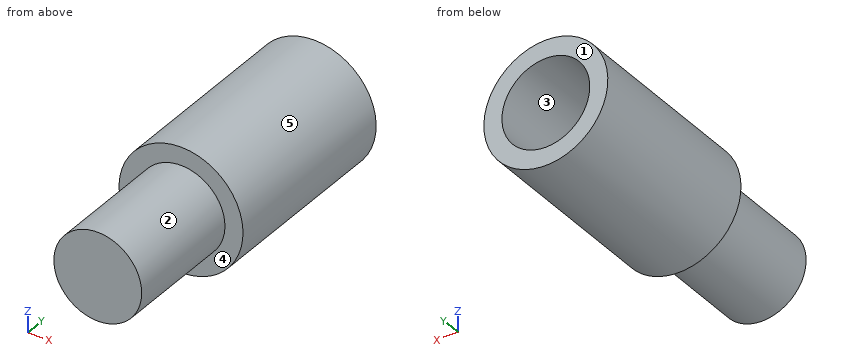
```python
from build123d import *

# Parameters (mm, degrees)
SKETCH1_R           = 12.7
BOSS_EXTRUDE1_DEPTH = 15
SKETCH2_R           = 9
BOSS_EXTRUDE2_DEPTH = 25
SKETCH3_R           = 12.7
SKETCH3_R_2         = 9
BOSS_EXTRUDE3_DEPTH = 25


with BuildPart() as part:
    # Sketch1 → Boss-Extrude1 (new body)
    with BuildSketch(Plane(origin=(0, 0, 0), x_dir=(1, 0, 0), z_dir=(0, 1, 0))):
        with Locations(Location((0, 0, 0), (0, 0, 270))):
            Circle(SKETCH1_R)
    extrude(amount=BOSS_EXTRUDE1_DEPTH)

    # Sketch2 → Boss-Extrude2 (add)
    with BuildSketch(Plane.XZ):
        with Locations(Location((0, 0, 0), (0, 0, 270))):
            Circle(SKETCH2_R)
    extrude(amount=BOSS_EXTRUDE2_DEPTH)

    # Sketch3 → Boss-Extrude3 (add)
    with BuildSketch(Plane(origin=(0, 15, 0), x_dir=(1, 0, 0), z_dir=(0, 1, 0))):
        with Locations(Location((0, 0, 0), (0, 0, 270))):
            Circle(SKETCH3_R)
        with Locations(Location((0, 0, 0), (0, 0, 90))):
            Circle(SKETCH3_R_2, mode=Mode.SUBTRACT)
    extrude(amount=BOSS_EXTRUDE3_DEPTH)


solid = part.part
```
The listing builds one solid part. Answer for the finished solid, in the listing's coordinates (mm). Face numbers are marked on the shaded views. A direction names the side the tool comes from. Coordinates: 2 decimals unless noted, no trailing zeros. Order: outer loops, then holes, each group sorted by start corner. A loop starts at its lowest first (then second) coordinate and runs counter-clockwise, first axis right, second up. Notation, with made-up numbers: M 22.5,-11 L 37.5,-11 A27 cw 37.5,23 Z; hole C 88.25,28 d6. An arc over 180 degrees is marked long. Answer as a JSON object with one key per item and string values. Group by question number.
1. Section C-C on y = 29.5 is taken. Write down the section's boundary in (x, z), then the cut area to 3 significant figures.
2. A tool of negligible diameter and unlimited length cuts with its end or side. For the marked faces 4 and 5, from which of +Z, -Z, +X, -X, +Y, -Y can it reach the whole face along a straight path? Write none if from no direction.
3. Straight lines are drawn through the part: line 1 (X direction, y = 31.75, z = 0); line 2 (Y direction, x = -10, z = -1.75); line 3 (Y direction, x = -4, z = -5.75). For each, find the intervals that lie inside material, in ascending order.
4. Section D-D on y = 13 is taken. Write down the section's boundary in (x, z).
5. Section B-B on z = 0 is taken. Write down the section's boundary in (x, y), then the cut area to 3 significant figures.
6. Flat-ended cylindrical pins translate along their axes: P1, Ø6, axis at y = 23.5, z = -6, coming from the -X side; P2, Ø4, axis at x = -2.5, y = 31, coming from the +Z side; P3, Ø1.5, axis at x = -7, z = -4, coming from the +Y side. Find the tip coordinate at first contact, or state that the pin passes through.
7. Determine the mould class of the marked faces 1, 2 and 3 for opening direction X: released by +X, released by -X, zero draft, split by the parting line, or undercut.
8. Section A-A on x = 0 is taken. Write down the section's boundary in (y, z).
Values follow:
{
 "1": {"outline": "C 0,0 d25.4; hole C 0,0 d18", "area": "252 mm2"},
 "2": {"face 4": "-Y", "face 5": "+Y, -Y"},
 "3": {"line 1": "-12.7 to -9, 9 to 12.7", "line 2": "0 to 40", "line 3": "-25 to 15"},
 "4": {"outline": "C 0,0 d25.4"},
 "5": {"outline": "M -12.7,0 L -9,0 L -9,-25 L 9,-25 L 9,0 L 12.7,0 L 12.7,40 L 9,40 L 9,15 L -9,15 L -9,40 L -12.7,40 Z", "area": "1,020 mm2"},
 "6": {"P1": "x = -12.34", "P2": "z = 12.69", "P3": "y = 15"},
 "7": {"face 1": "zero draft", "face 2": "split by the parting line", "face 3": "undercut"},
 "8": {"outline": "M -25,-9 L 0,-9 L 0,-12.7 L 40,-12.7 L 40,-9 L 15,-9 L 15,9 L 40,9 L 40,12.7 L 0,12.7 L 0,9 L -25,9 Z"}
}
